Autodesk Inventor part; units mm, degrees
ref_plane "YZ Plane" through (0, 0, 0) normal (1, 0, 0) x (0, 1, 0)
ref_plane "XZ Plane" through (0, 0, 0) normal (0, 1, 0) x (-1, 0, 0)
ref_plane "XY Plane" through (0, 0, 0) normal (0, 0, 1) x (1, 0, 0)
sketch "Sketch1" plane through (0, 0, 0) normal (0, 1, 0) x (-1, 0, 0)
  line L0 (0, 0) -> (-600, 0)
  line L1 (-600, 0) -> (-600, -20)
  line L2 (-600, -20) -> (0, -20)
  line L3 (0, -20) -> (0, 0)
  dimension "d0" = 600
  dimension "d1" = 20
extrude "Extrusion1" add sketch "Sketch1" along normal blind 2
sketch "Sketch2" plane through (0, 2, 0) normal (0, 1, 0) x (1, 0, 0)
  line L0 (0, 0) -> (600, 0)
  line L1 (600, 0) -> (600, 2)
  line L2 (600, 2) -> (0, 2)
  line L3 (0, 2) -> (0, 0)
  dimension "d4" = 600
  dimension "d5" = 2
extrude "Extrusion2" add sketch "Sketch2" along normal blind 18
hole "Hole1" at (60, 10, 0) direction (0, 0, -1) diameter 5.5 end through all
pattern_linear "Rectangular Pattern1" count 6 spacing 90 along (1, 0, 0) of "Hole1"
ref_plane "Work Plane1" through (450, 2, -2) normal (0, 0.7071, 0.7071) x (1, 0, 0)
mirror "Mirror1" about plane through (450, 2, -2) normal (0, 0.7071, 0.7071) of "Hole1", "Rectangular Pattern1"
properties part number "Lbarx2" material "Aluminum 6061"
Work out the finished part from the listing and answer in its coordinate system (mm). A direction names the side the tool comes from. Give positions to 0.01 mm unless a question says otherwise; leave off trailing zeros. Loops run counter-clockwise (first coordinate to the right, second up) from the corner with the lowest first, then second, coordinate; pieces in that order, holes last. Notation, with made-up numbers: (83, 49) - (119, 49) arc R26 ccw to (119, 86) - close; hole circle Ø7 at (-4, 80.25). An arc over 180 degrees is marked (long way). Answer in a Markdown table with one row per item. Add a question column.
Q1. A tool of negligible diameter and unlimited length cuts with its end or side. For faces 1 (the flat face through (304, 2, -11)), 2 (the flat face through (600, 5.5, -1.8)), from which of +Z, -Z, +X, -X, +Y, -Y can it reach the whole face along a straight path? Write none if from no direction.
Q2. The part is cut by section A-A (x = 547). Determine the outline of the cut face in (y, z).
Q3. Consider line 1 along Y through (x, z) = (330, -1.1); line 2 along Z through (x, y) = (510, 0.8); line 3 along Y through (x, z) = (545, -14.25). Determine where each line is inside the solid, lowest interval first.
Q4. Each of these flat-tipped pins is pushed along its axis until it touches: P1, Ø7, axis at x = 240, z = -10, coming from the +Y side; P2, Ø9, axis at x = 60, y = 10, coming from the -Z side. Where does it stop, or does it pass through?
Solution:
| question | item | result |
|---|---|---|
| 1 | face 1 | -Z, +X, -X, +Y |
| 1 | face 2 | +Z, -Z, +X, +Y, -Y |
| 2 | outline | (0, -20) - (2, -20) - (2, -2) - (20, -2) - (20, 0) - (0, 0) - close |
| 3 | line 1 | y = 0 to 7.25, 12.75 to 20 |
| 3 | line 2 | z = -20 to -12.75, -7.25 to 0 |
| 3 | line 3 | y = 0 to 2 |
| 4 | P1 | stops at y = 2 |
| 4 | P2 | stops at z = -2 |
